Work out the finished part from the listing and answer in its coordinate system (mm). A direction names the side the tool comes from. Give positions to 0.01 mm unless a question says otherwise; leave off trailing zeros. Write each loop counter-clockwise with the first axis right and the second up, starting at its lowest first coordinate (ties: lowest second). Pieces come first, ordered by that corner, then holes. Notation, with made-up numbers: (-5.75, 88.5) - (18.25, 88.5) arc R18 cw to (18.25, 120.5) - close; hole circle Ø10 at (73, 57). An arc over 180 degrees is marked (long way). Write each question's results on one line, items separated by ' | '. Start each with the question number.
from build123d import *

# Parameters (mm, degrees)
SKETCH1_R           = 5
BOSS_EXTRUDE1_DEPTH = 14
SKETCH2_W           = 1
SKETCH2_H           = 15.34768378
CUT_EXTRUDE1_DEPTH  = 15
SKETCH3_R           = 2.75
CUT_EXTRUDE2_DEPTH  = 7


with BuildPart() as part:
    # Sketch1 → Boss-Extrude1 (new body)
    with BuildSketch(Plane.XY):
        Polygon((9, 12.8), (-9, 12.8), (-9, -14), (-21, -14), (-21, -20), (21, -20), (21, -14), (9, -14), align=None)
        Circle(SKETCH1_R, mode=Mode.SUBTRACT)
    extrude(amount=BOSS_EXTRUDE1_DEPTH)

    # Sketch2 → Cut-Extrude1 (cut, through all)
    with BuildSketch(Plane.XY.offset(14)):
        with Locations((0, 7.003057882)):
            Rectangle(SKETCH2_W, SKETCH2_H)
    extrude(amount=-CUT_EXTRUDE1_DEPTH, mode=Mode.SUBTRACT)

    # Sketch3 → Cut-Extrude2 (cut, through all)
    with BuildSketch(Plane(origin=(0, -14, 0), x_dir=(1, 0, 0), z_dir=(0, 1, 0))):
        with Locations((-16, -7)):
            Circle(SKETCH3_R)
        with Locations((16, -7)):
            Circle(SKETCH3_R)
    extrude(amount=-CUT_EXTRUDE2_DEPTH, mode=Mode.SUBTRACT)


solid = part.part
Q1. A tool of negligible diameter and unlimited length cuts with its end or side. For faces 4 (the flat face through (0.5, 9, 7)), 5 (the flat face through (9, -1, 7)), 6 (the flat face through (-9, 0, 7)), from which of +Z, -Z, +X, -X, +Y, -Y can it reach the whole face along a straight path? Write none if from no direction.
Q2. A cutting plane is placed at D-D, the plane z = 8. Write down the section's boundary in (x, y).
Q3. A cutting plane is placed at A-A, the plane x = 16. Write down the section's boundary in (y, z), and give its area (3 significant figures).
Q4. A cutting plane is placed at B-B, the plane y = 0. Write down the section's boundary in (x, z), and give its area (3 significant figures).
Q5. Given pin 1 (3.5 mm diameter, centred on x = 14.5, z = 5.5, fed in from +Y); pin 2 (4 mm diameter, centred on y = -2.5, z = 5.5, fed in from -X); pin 3 (4 mm diameter, centred on y = 1.5, z = 7, fed in from +X), each flat-ended and moving along its own axis, determine where each tip first touches the part or whether it passes through.
Q6. A cutting plane is placed at C-C, the plane z = 3.5. Write down the section's boundary in (x, y), and give its area (3 significant figures).
Q7. Consider L1, parallel to X at y = -15.9, z = 7; L2, parallel to X at y = 10.5, z = 1.75; L3, parallel to Z at x = -16, y = -16.4. Determine where each line is inside the solid, lowest interval first.
Q8. The mould has two halves that part along Y. Classify faces 1 (the flat face through (0, -20, 7)), 2 (the cylindrical face through (0, -5, 7)), 3 (the flat face through (-0.5, 9, 7)): pulls with the +Y half, pulls with the -Y half, needs draft (parallel to the pull), parting line crosses it, or undercut.
Result:
1) face 4: +Z, -Z, +Y | face 5: +Z, -Z, +X, +Y | face 6: +Z, -Z, -X, +Y
2) outline: (-21, -20) - (-18.56, -20) - (-18.56, -14) - (-21, -14) - close; (-13.44, -20) - (13.44, -20) - (13.44, -14) - (9, -14) - (9, 12.8) - (0.5, 12.8) - (0.5, 4.97) arc R5 cw (long way) to (-0.5, 4.97) - (-0.5, 12.8) - (-9, 12.8) - (-9, -14) - (-13.44, -14) - close; (18.56, -20) - (21, -20) - (21, -14) - (18.56, -14) - close
3) outline: (-20, 0) - (-14, 0) - (-14, 4.25) - (-20, 4.25) - close; (-20, 9.75) - (-14, 9.75) - (-14, 14) - (-20, 14) - close | area: 51.0 mm2
4) outline: (-9, 0) - (-5, 0) - (-5, 14) - (-9, 14) - close; (5, 0) - (9, 0) - (9, 14) - (5, 14) - close | area: 112 mm2
5) pin 1: stops at y = -14 | pin 2: stops at x = -9 | pin 3: stops at x = 9
6) outline: (-21, -20) - (21, -20) - (21, -14) - (9, -14) - (9, 12.8) - (0.5, 12.8) - (0.5, 4.97) arc R5 cw (long way) to (-0.5, 4.97) - (-0.5, 12.8) - (-9, 12.8) - (-9, -14) - (-21, -14) - close | area: 648 mm2
7) L1: x = -21 to -18.75, -13.25 to 13.25, 18.75 to 21 | L2: x = -9 to -0.5, 0.5 to 9 | L3: z = 0 to 4.25, 9.75 to 14
8) face 1: pulls with the -Y half | face 2: undercut | face 3: needs draft
